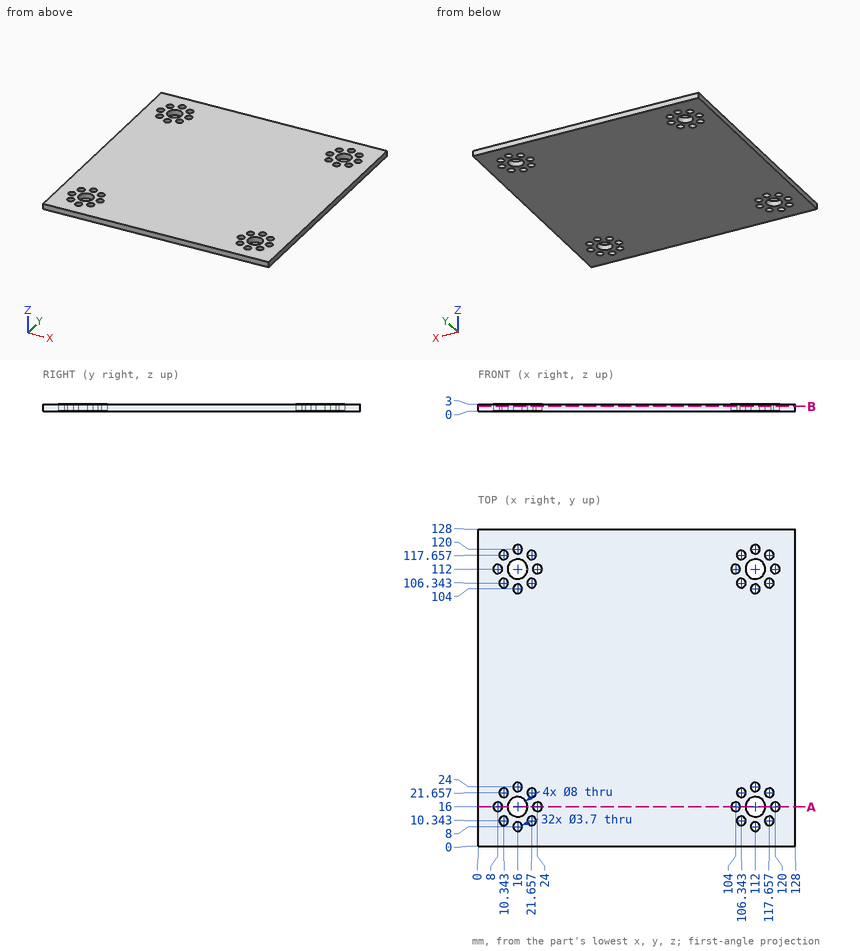
Verification items for this drawing (mm, ordinates from the low corner). Give positions to 0.01 mm unless a question says otherwise; leave off trailing zeros. Write each loop counter-clockwise with the first axis right and the second up, starting at its lowest first coordinate (ties: lowest second). Pieces come first, ordered by that corner, then holes.
1) Gauge pin test, flat end, axial feed: pin 1 (3.5 mm diameter, centred on x = 16, y = 104, fed in from -Z). Record the tip position at first contact, or that the pin passes through.
2) Section check B-B, the plane z = 2. State how many separate pieces and enclosed holes the cut face has, and give its area (3 significant figures).
3) Section check A-A, the plane y = 16. Record the boundary of the cut face in (x, z).
4) Material ranges on L1, parallel to X at y = 8, z = 1.05; L2, parallel to Y at x = 116.5, z = 2.2, recorded low to high.
Computed:
1. pin 1: passes through
2. separate pieces: 1
2. enclosed holes: 36
2. area: 15,800 mm2
3. outline: (0, 0) - (6.15, 0) - (6.15, 3) - (0, 3) - close; (9.85, 0) - (12, 0) - (12, 3) - (9.85, 3) - close; (20, 0) - (22.15, 0) - (22.15, 3) - (20, 3) - close; (25.85, 0) - (102.15, 0) - (102.15, 3) - (25.85, 3) - close; (105.85, 0) - (108, 0) - (108, 3) - (105.85, 3) - close; (116, 0) - (118.15, 0) - (118.15, 3) - (116, 3) - close; (121.85, 0) - (128, 0) - (128, 3) - (121.85, 3) - close
4. L1: x = 0 to 14.15, 17.85 to 110.15, 113.85 to 128
4. L2: y = 0 to 8.9, 11.79 to 20.21, 23.1 to 104.9, 107.79 to 116.21, 119.1 to 128
